```python
from build123d import *

# Parameters (mm, degrees)
SKETCH_R        = 6.05
SKETCH_W        = 19.9
SKETCH_H        = 6.4
PAD_DEPTH       = 10
SKETCH002_W     = 3
SKETCH002_H     = 6.9
POCKET001_DEPTH = 12
SKETCH003_R     = 2.25
POCKET_DEPTH    = 6
SKETCH004_R     = 2.25
POCKET002_DEPTH = 25.901


with BuildPart() as part:
    # Sketch → Pad (new body)
    with BuildSketch(Plane.XY):
        with BuildLine():
            ThreePointArc((12.95, 0), (0, 12.95), (-12.95, 0))
            Line((-12.95, 0), (-12.95, -30.2))
            Line((-12.95, -30.2), (12.95, -30.2))
            Line((12.95, -30.2), (12.95, 0))
        make_face()
        Circle(SKETCH_R, mode=Mode.SUBTRACT)
        with Locations((0, -25)):
            Rectangle(SKETCH_W, SKETCH_H, mode=Mode.SUBTRACT)
    extrude(amount=PAD_DEPTH)

    # Sketch002 → Pocket001 (cut)
    with BuildSketch(Plane.XY.offset(10)):
        with Locations((-8.5, 0)):
            Rectangle(SKETCH002_W, SKETCH002_H)
    extrude(amount=-POCKET001_DEPTH, mode=Mode.SUBTRACT)

    # Sketch003 → Pocket (cut, symmetric)
    with BuildSketch(Plane.YZ.offset(-9.95)):
        with Locations((0, 5)):
            Circle(SKETCH003_R)
    extrude(amount=POCKET_DEPTH, both=True, mode=Mode.SUBTRACT)

    # Sketch004 → Pocket002 (cut, through all)
    with BuildSketch(Plane.YZ.offset(12.95)):
        with Locations((0, 5)):
            Circle(SKETCH004_R)
    extrude(amount=-POCKET002_DEPTH, mode=Mode.SUBTRACT)


solid = part.part
```
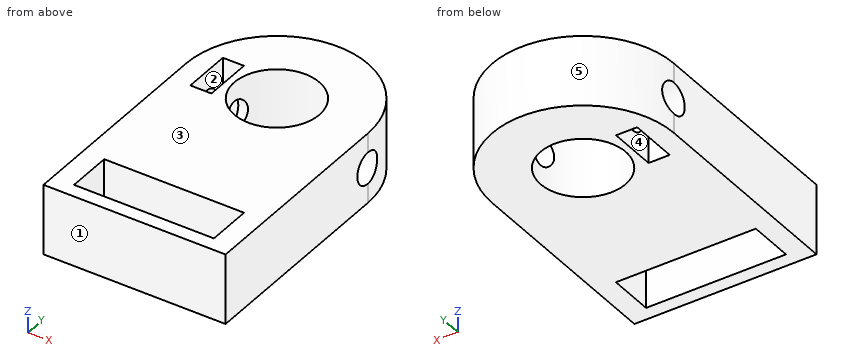
Could you check a few things on this model? Use its own coordinates, in mm. Face numbers are marked on the shaded views. A direction names the side the tool comes from. Round coordinates to 2 decimals unless told otherwise and drop trailing zeros. Loops run counter-clockwise (first coordinate to the right, second up) from the corner with the lowest first, then second, coordinate; pieces in that order, holes last. Notation, with made-up numbers: (86.5, -20) - (134.5, -20) arc R20 ccw to (134.5, 18) - close; hole circle Ø3 at (32.5, -22). An arc over 180 degrees is marked (long way). Answer in a Markdown table with one row per item. Add a question column.
(1) For the marked faces 1 and 2, which set-ups out of +Z, -Z, +X, -X, +Y, -Y let a thin tool reach every point of the face, with its end or its side?
(2) I'm going to push flat-ended pins straight in: pin 1 (11 mm diameter, centred on x = 0, y = 0, fed in from +Z); pin 2 (0.9 mm diameter, centred on x = -8, z = 4, fed in from +Y); pin 3 (1.5 mm diameter, centred on y = 7, z = 7.5, fed in from -X). Where does each tip first touch, or does it pass through?
(3) If we section it at D-D (y = -3): Please give me the cut outline in (x, z).
(4) I need wall thicknesses on line 1 along Y through (x, z) = (0, 7.5); line 2 along X through (y, z) = (1.5, 7.25); line 3 along Y through (x, z) = (-6.6, 5). Which ranges of each line are inside material? Lowest first, please.
(5) If we mould it in two halves opening along Y, with no side actions, what happens to the marked faces 3, 4 and 5? For each: pulls with the +Y half, pulls with the -Y half, needs draft (parallel to the pull), parting line crosses it, or undercut.
(6) If we section it at C-C (z = 5): Please give me the cut outline in (x, y), plus the area to 3 significant figures.
(7) If we section it at A-A (y = -24.5): Please give me the cut outline in (x, z), plus the area to 3 significant figures.
(8) If we section it at B-B (x = 0): Please give me the cut outline in (y, z).
Model answer:
| question | item | result |
|---|---|---|
| 1 | face 1 | +Z, -Z, +X, -X, -Y |
| 1 | face 2 | +Z, -Z |
| 2 | pin 1 | passes through |
| 2 | pin 2 | stops at y = 10.52 |
| 2 | pin 3 | stops at x = -11.34 |
| 3 | outline | (-12.95, 0) - (-10, 0) - (-10, 10) - (-12.95, 10) - close; (-7, 0) - (-5.25, 0) - (-5.25, 10) - (-7, 10) - close; (5.25, 0) - (12.95, 0) - (12.95, 10) - (5.25, 10) - close |
| 4 | line 1 | y = -30.2 to -28.2, -21.8 to -6.05, 6.05 to 12.95 |
| 4 | line 2 | x = -12.86 to -10, -7 to -5.86, 5.86 to 12.86 |
| 4 | line 3 | y = -30.2 to -28.2, -21.8 to -2.25, 2.25 to 11.14 |
| 5 | face 3 | needs draft |
| 5 | face 4 | undercut |
| 5 | face 5 | pulls with the +Y half |
| 6 | outline | (-12.95, -30.2) - (12.95, -30.2) - (12.95, -2.25) - (5.62, -2.25) arc R6.05 cw to (-5.62, -2.25) - (-7, -2.25) - (-7, -3.45) - (-10, -3.45) - (-10, -2.25) - (-12.95, -2.25) - close; (-12.75, 2.25) - (-10, 2.25) - (-10, 3.45) - (-7, 3.45) - (-7, 2.25) - (-5.62, 2.25) arc R6.05 cw to (5.62, 2.25) - (12.75, 2.25) arc R12.95 ccw to start; hole (-9.95, -28.2) - (9.95, -28.2) - (9.95, -21.8) - (-9.95, -21.8) - close |
| 6 | area | 733 mm² |
| 7 | outline | (-12.95, 0) - (-9.95, 0) - (-9.95, 10) - (-12.95, 10) - close; (9.95, 0) - (12.95, 0) - (12.95, 10) - (9.95, 10) - close |
| 7 | area | 60.0 mm² |
| 8 | outline | (-30.2, 0) - (-28.2, 0) - (-28.2, 10) - (-30.2, 10) - close; (-21.8, 0) - (-6.05, 0) - (-6.05, 10) - (-21.8, 10) - close; (6.05, 0) - (12.95, 0) - (12.95, 10) - (6.05, 10) - close |
